Autodesk Inventor part; units mm, degrees
ref_plane "YZ Plane" through (0, 0, 0) normal (1, 0, 0) x (0, 1, 0)
ref_plane "XZ Plane" through (0, 0, 0) normal (0, 1, 0) x (-1, 0, 0)
ref_plane "XY Plane" through (0, 0, 0) normal (0, 0, 1) x (1, 0, 0)
sketch "Sketch1" plane through (0, 0, 0) normal (0, 1, 0) x (-1, 0, 0)
  circle A0 centre (0, 0) radius 15.875
  line L0 (0, 0) -> (12.3952, 0)
  circle A1 centre (12.3952, 0) radius 1.905
  circle A2 centre (0, 0) radius 8.89
  circle A3 centre (-6.1976, 10.7346) radius 1.905
  circle A4 centre (-6.1976, -10.7346) radius 1.905
  dimension "d0" = 31.75
  dimension "d1" = 12.3952
  dimension "d2" = 3.81
  dimension "d3" = 17.78
  dimension "d6" = 360
extrude "Extrusion1" add sketch "Sketch1" along normal blind 4.445
properties part number "SmallSpoolExpander" material "ABS Plastic"
Check sheet for the modelled part. Datum: model origin and axes. Units: mm. Round coordinates to 2 decimals unless told otherwise and drop trailing zeros. Write each loop counter-clockwise with the first axis right and the second up, starting at its lowest first coordinate (ties: lowest second). Pieces come first, ordered by that corner, then holes. Notation, with made-up numbers: (80, -24) - (103, -24) arc R23 cw to (103, 5) - close; hole circle Ø7 at (-12, 65). An arc over 180 degrees is marked (long way). Return JSON: item names as keys, results as strings.
Q1. Scan lines: L1, parallel to Z at x = 0, y = 1.4 (3 decimals); L2, parallel to X at y = 4.15, z = 1; L3, parallel to Z at x = -1, y = 2.85. Record each from-to range of solid material in increasing order. Write a range as from..to.
Returned:
{"L1": "z = -15.875..-8.89, 8.89..15.875", "L2": "x = -15.84..-14.02, -10.77..-8.83, 8.83..15.84", "L3": "z = -15.84..-8.83, 8.83..15.84"}
Q2. Draft check along X on faces 1 (the cylindrical face through (8.1, 2.19, 10.65)), 2 (the flat face through (-7, 4.445, -7)), 3 (the cylindrical face through (3.441, 2.191, 15.497)). Enter one of: released by +X, released by -X, zero draft, split by the parting line, or undercut.
Returned:
{"face 1": "undercut", "face 2": "zero draft", "face 3": "split by the parting line"}
Q3. Cross-section at D-D (y = 2). Record the boundary of the cut face in (x, z) (3 decimals).
Returned:
{"outline": "circle Ø31.75 at (0, 0); hole circle Ø3.81 at (-12.395, 0); hole circle Ø17.78 at (0, 0); hole circle Ø3.81 at (6.198, -10.735); hole circle Ø3.81 at (6.198, 10.735)"}
Q4. Cross-section at B-B (x = 0). Record the boundary of the cut face in (y, z) (3 decimals).
Returned:
{"outline": "(0, -15.875) - (4.445, -15.875) - (4.445, -8.89) - (0, -8.89) - close; (0, 8.89) - (4.445, 8.89) - (4.445, 15.875) - (0, 15.875) - close"}
Q5. Cross-section at C-C (z = 5). Record the boundary of the cut face in (x, y) (3 decimals).
Returned:
{"outline": "(-15.067, 0) - (-7.351, 0) - (-7.351, 4.445) - (-15.067, 4.445) - close; (7.351, 0) - (15.067, 0) - (15.067, 4.445) - (7.351, 4.445) - close"}
Q6. Depth check by flat-ended pin: P1, Ø1.5, axis at y = 1, z = -11, coming from the +X side; P2, Ø1.5, axis at x = 6, y = 2.5, coming from the -Z side. Enter the tip coordinate at first touch or a pass-through.
Returned:
{"P1": "stops at x = 12.12", "P2": "stops at z = -14.98"}
Q7. Cross-section at A-A (z = 0). Record the boundary of the cut face in (x, y) (3 decimals).
Returned:
{"outline": "(-15.875, 0) - (-14.3, 0) - (-14.3, 4.445) - (-15.875, 4.445) - close; (-10.49, 0) - (-8.89, 0) - (-8.89, 4.445) - (-10.49, 4.445) - close; (8.89, 0) - (15.875, 0) - (15.875, 4.445) - (8.89, 4.445) - close"}
